```python
from build123d import *

# Parameters (mm, degrees)
F0_W     = 76.2
F0_H     = 76.2
F0_R     = 19.05
F1_DEPTH = 25.4


# Not quite as in the source:
# - the program builds the solid bodies; features that only make, move or delete a surface that nothing else refers to are left out


with BuildPart() as f1:
    # F0 (on Front) → F1 (new body)
    with BuildSketch(Plane.XZ):
        Rectangle(F0_W, F0_H)
        Circle(F0_R, mode=Mode.SUBTRACT)
    extrude(amount=F1_DEPTH)


solid = f1.part
```
The listing builds one solid part. Answer for the finished solid, in the listing's coordinates (mm). Round coordinates to 2 decimals unless told otherwise and drop trailing zeros. Order: outer loops, then holes, each group sorted by start corner. A loop starts at its lowest first (then second) coordinate and runs counter-clockwise, first axis right, second up. Notation, with made-up numbers: (14, -2) -> (31, -2) arc R19 ccw to (31, 6) -> close; hole circle Ø7 at (1.5, 89.25). An arc over 180 degrees is marked (long way). Answer as CSV lines item,"result". Start each with the question number.
(1) The part is cut by section B-B (x = 0). Determine the outline of the cut face in (y, z), then the cut area to 3 significant figures.
(2) The part is cut by section C-C (y = -11). Determine the outline of the cut face in (x, z), then the cut area to 3 significant figures.
(3) The part is cut by section A-A (z = 0). Determine the outline of the cut face in (x, y).
(4) For a pull along Z with two mould halves and no side action, classify faces 1 (the face through (-9, -25.4, 17)), 2 (the face through (-1, -13, -38.1)), 3 (the face through (-15.12, -12.52, -11.59)) as +Z half, -Z half, draft (parallel to the pull), parting line (faces both ways), or undercut.
(5) A flat-ended cylindrical pin translates along its axis: pin 1 Ø23 at (x, z) = (0, 0) entering from +Y. Find the tip coordinate at first contact, or state that the pin passes through.
(6) Find the intervals of material crossed by probe 1 along Z at (x, y) = (0, -13.75); probe 2 along X at (y, z) = (-14.5, -0.5); probe 3 along Z at (x, y) = (16, -18.75), in increasing order. Write a range as from..to.
Evaluation:
1,outline,"(-25.4, -38.1) -> (0, -38.1) -> (0, -19.05) -> (-25.4, -19.05) -> close; (-25.4, 19.05) -> (0, 19.05) -> (0, 38.1) -> (-25.4, 38.1) -> close"
1,area,"968 mm²"
2,outline,"(-38.1, -38.1) -> (38.1, -38.1) -> (38.1, 38.1) -> (-38.1, 38.1) -> close; hole circle Ø38.1 at (0, 0)"
2,area,"4,670 mm²"
3,outline,"(-38.1, -25.4) -> (-19.05, -25.4) -> (-19.05, 0) -> (-38.1, 0) -> close; (19.05, -25.4) -> (38.1, -25.4) -> (38.1, 0) -> (19.05, 0) -> close"
4,face 1,"draft"
4,face 2,"-Z half"
4,face 3,"undercut"
5,pin 1,"through"
6,probe 1,"-38.1..-19.05, 19.05..38.1"
6,probe 2,"-38.1..-19.04, 19.04..38.1"
6,probe 3,"-38.1..-10.34, 10.34..38.1"
